For this review, use the dimensioned drawing (mm, ordinates from the lowest corner) and the shaded views. Give positions to 0.01 mm unless a question says otherwise; leave off trailing zeros. Loops run counter-clockwise (first coordinate to the right, second up) from the corner with the lowest first, then second, coordinate; pieces in that order, holes last. Notation, with made-up numbers: M 19,46 L 61,46 A24 cw 61,64 Z; hole C 58.25,71 d7. An arc over 180 degrees is marked long. Use CSV: the item, a comma, the result in double quotes. Start each with the question number.
1. Insertion check: P1, Ø1.2, axis at y = 1.5, z = 122, coming from the +X side; P2, Ø2, axis at x = 482, y = 2.5, coming from the +Z side; P3, Ø1.5, axis at y = 1, z = 34, coming from the +X side. Each pin has a flat end and moves straight along its axis. Give the tip position at first contact, or say it passes through.
2. Take a section at C-C, the plane z = 31.5. Write out the cut boundary in (x, y).
3. Take a section at A-A, the plane y = 1.6. Write out the cut boundary in (x, z).
4. To check wall thickness, follow line 1 (X direction, y = 0.6, z = 111); line 2 (Z direction, x = 96, y = 0.45); line 3 (X direction, y = 2.5, z = 58.5). State the ranges of each line that lie inside material, in increasing order. Write a range as [from, to].
5. Take a section at B-B, the plane z = 135. Write out the cut boundary in (x, y), and give its area (3 significant figures).
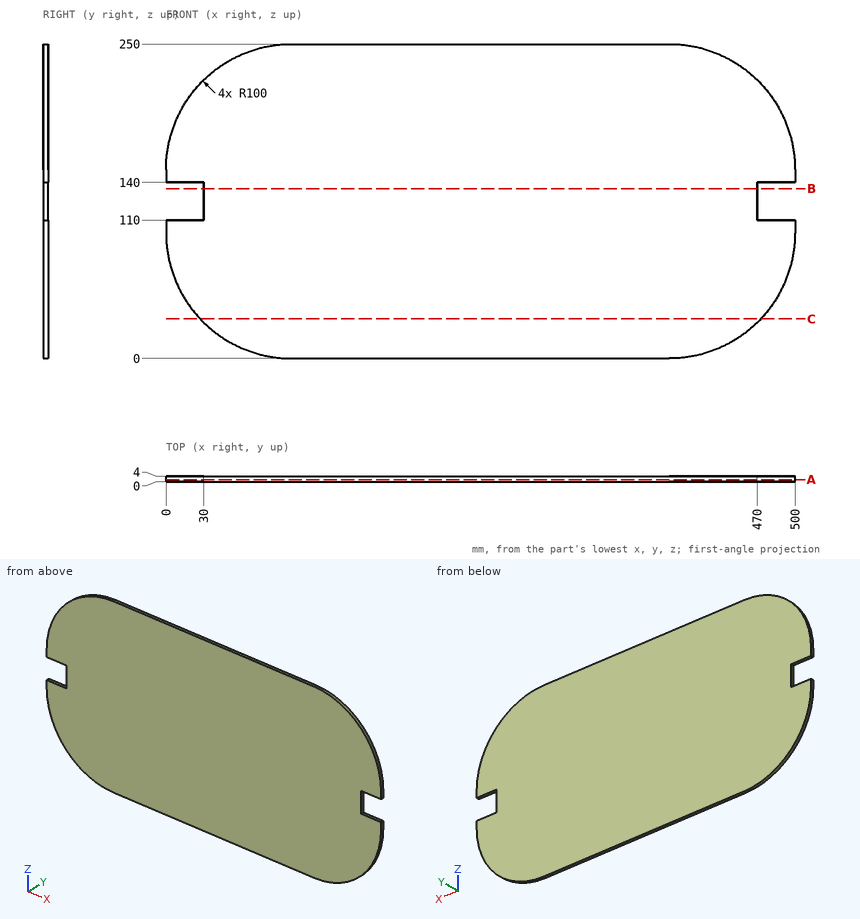
Result set:
1,P1,"x = 470"
1,P2,"z = 208.64"
1,P3,"x = 475.78"
2,outline,"M 27.15,0 L 472.85,0 L 472.85,4 L 27.15,4 Z"
3,outline,"M 0,100 A100 ccw 100,0 L 400,0 A100 ccw 500,100 L 500,110 L 470,110 L 470,140 L 500,140 L 500,150 A100 ccw 400,250 L 100,250 A100 ccw 0,150 L 0,140 L 30,140 L 30,110 L 0,110 Z"
4,line 1,"[30, 470]"
4,line 2,"[0.08, 249.92]"
4,line 3,"[9.02, 490.98]"
5,outline,"M 30,0 L 470,0 L 470,4 L 30,4 Z"
5,area,"1,760 mm2"
